Autodesk Inventor part; units mm, degrees
ref_plane "YZ Plane" through (0, 0, 0) normal (1, 0, 0) x (0, 1, 0)
ref_plane "XZ Plane" through (0, 0, 0) normal (0, 1, 0) x (-1, 0, 0)
ref_plane "XY Plane" through (0, 0, 0) normal (0, 0, 1) x (1, 0, 0)
sketch "Sketch1" plane through (0, 0, 0) normal (0, 0, 1) x (1, 0, 0)
  arc A0 (967.6192, 924.0732) -> (967.7873, 1075.2272) centre (902.2196, 999.723) ccw
  arc A1 (983.2683, 893.0126) -> (983.4428, 1106.3006) centre (902.2196, 999.723) ccw
  line L0 (965.7611, 927.7614) -> (985.0977, 889.3816)
  line L1 (966.6908, 925.9161) -> (1011.6908, 925.9161) construction
  arc A2 (985.0977, 889.3816) -> (985.2727, 1109.9327) centre (902.2196, 999.723) ccw
  line L2 (965.9281, 1071.5369) -> (985.2727, 1109.9327)
  arc A3 (965.7611, 927.7614) -> (965.9281, 1071.5369) centre (902.2196, 999.723) ccw
  line L3 (977.4986, 940.149) -> (980.6353, 937.6667)
  point P0 (0, 0)
  point P1 (983.9681, 893.1)
  point P2 (990.6031, 1100.4422)
  point P3 (968.1775, 1074.8866)
  dimension "d28" = 100
  dimension "d33" = 63.26
  dimension "d34" = 4
  dimension "d40" = 4
  dimension "d41" = 4
extrude "Extrusion6" add sketch "Sketch1" along normal blind 5
extrude "Extrusion7" add sketch "Sketch1" along normal blind 17 contours L3 A3 L2 A0 | A1 L2 A2 L0
sketch "Sketch5" plane through (0, 0, 5) normal (0, 0, 1) x (1, 0, 0)
  arc A0 (965.7611, 927.7614) -> (977.4986, 940.149) centre (902.2196, 999.723) ccw
  line L0 (965.7611, 927.7614) -> (970.2605, 918.8308)
  line L1 (965.7611, 927.7614) -> (983.2683, 893.0126)
  line L2 (977.4986, 940.149) -> (985.1361, 933.6938)
  arc A1 (965.7611, 927.7614) -> (977.4986, 940.149) centre (902.2196, 999.723) ccw
  arc A2 (965.7611, 927.7614) -> (974.9009, 937.006) centre (902.2196, 999.723) ccw
  line L3 (974.9009, 937.006) -> (982.5384, 930.5509)
  arc A3 (970.2605, 918.8308) -> (982.5384, 930.5509) centre (950.8165, 951.4915) ccw
  point P0 (0, 0)
  dimension "d42" = 10
  dimension "d43" = 10
  dimension "d46" = 13
  dimension "d47" = 10
extrude "Extrusion8" cut sketch "Sketch5" along normal through all both and the other way through all
sketch "Sketch6" plane through (0, 0, 5) normal (0, 0, 1) x (1, 0, 0)
  arc A0 (974.9009, 937.006) -> (965.9281, 1071.5369) centre (902.2196, 999.723) ccw
  arc A1 (985.0977, 889.3816) -> (985.2727, 1109.9327) centre (902.2196, 999.723) ccw
  line L0 (985.8441, 1046.8712) -> (1027.8759, 1046.8712) construction
  line L1 (985.2727, 1109.9327) -> (965.9281, 1071.5369)
  line L2 (965.9281, 1071.5369) -> (985.2727, 1109.9327)
  arc A2 (985.8441, 1046.8712) -> (965.9281, 1071.5369) centre (902.2196, 999.723) ccw
  arc A3 (1007.3627, 1089.1038) -> (985.2727, 1109.9327) centre (902.2196, 999.723) ccw
  line L3 (985.8441, 1046.8712) -> (1007.3627, 1089.1038)
  point P0 (0, 0)
  dimension "d51" = 63
extrude "Extrusion9" cut sketch "Sketch6" along normal through all both and the other way through all
sketch "Sketch7" plane through (0, 0, 5) normal (0, 0, 1) x (1, 0, 0)
  arc A0 (977.4782, 940.1232) -> (985.8441, 1046.8712) centre (902.2196, 999.723) ccw
  arc A1 (980.614, 937.6399) -> (988.005, 1051.1123) centre (902.2196, 999.723) ccw
  arc A2 (974.9009, 937.006) -> (985.8441, 1046.8712) centre (902.2196, 999.723) ccw
  line L0 (985.8441, 1046.8712) -> (988.005, 1051.1123)
  line L1 (985.8441, 1046.8712) -> (1007.3627, 1089.1038)
  line L2 (993.2753, 1030.1346) -> (996.6034, 1032.7639)
  point P0 (0, 0)
  dimension "d52" = 4
extrude "Extrusion10" cut sketch "Sketch7" along normal through all both and the other way through all
sketch "Sketch8" plane through (0, 0, 17) normal (0, 0, 1) x (1, 0, 0)
  arc A0 (983.2683, 893.0126) -> (1005.3901, 1085.2324) centre (902.2196, 999.723) ccw
  arc A1 (1014.3006, 1073.1658) -> (1005.3901, 1085.2324) centre (902.2196, 999.723) ccw
  line L0 (988.005, 1051.1123) -> (1007.3627, 1089.1038)
  line L1 (1005.3901, 1085.2324) -> (1007.3627, 1089.1038)
  line L2 (1014.3006, 1073.1658) -> (1017.6463, 1075.3581)
  arc A2 (985.0977, 889.3816) -> (1007.3627, 1089.1038) centre (902.2196, 999.723) ccw
  arc A3 (1017.6463, 1075.3581) -> (1007.3627, 1089.1038) centre (902.2196, 999.723) ccw
  point P0 (0, 0)
  dimension "d55" = 15
  dimension "d56" = 4
  dimension "d57" = 138
extrude "Extrusion11" cut sketch "Sketch8" against normal blind 12
sketch "Sketch10" plane through (0, 0, 5) normal (0, 0, 1) x (1, 0, 0)
  line L0 (993.2753, 1030.1346) -> (996.6034, 1032.7639)
  arc A0 (996.6034, 1032.7639) -> (988.005, 1051.1123) centre (902.2196, 999.723) ccw
  line L1 (988.005, 1051.1123) -> (1007.3627, 1089.1038)
  arc A1 (1017.6463, 1075.3581) -> (1007.3627, 1089.1038) centre (902.2196, 999.723) ccw
  line L2 (1014.3006, 1073.1658) -> (1017.6463, 1075.3581)
  arc A2 (983.2683, 893.0126) -> (1014.3006, 1073.1658) centre (902.2196, 999.723) ccw
  line L3 (983.2683, 893.0126) -> (970.2605, 918.8308)
  arc A3 (970.2605, 918.8308) -> (982.5384, 930.5509) centre (950.8165, 951.4915) ccw
  line L4 (982.5384, 930.5509) -> (974.9009, 937.006)
  arc A4 (974.9009, 937.006) -> (977.4986, 940.149) centre (902.2196, 999.723) ccw
  arc A5 (977.4986, 940.149) -> (993.2753, 1030.1346) centre (902.2196, 999.723) ccw
  arc A6 (980.6353, 937.6667) -> (996.6034, 1032.7639) centre (902.2196, 999.723) ccw
  line L5 (977.4986, 940.149) -> (980.6353, 937.6667)
  arc A7 (985.0977, 889.3816) -> (1017.6463, 1075.3581) centre (902.2196, 999.723) ccw
  line L6 (985.0977, 889.3816) -> (983.2683, 893.0126)
  line L7 (970.2605, 918.8308) -> (988.005, 1051.1123)
  line L8 (977.3926, 1032.2651) -> (974.8751, 1035.6786)
  arc A8 (988.005, 1051.1123) -> (974.8751, 1035.6786) centre (1057.2145, 978.9317) ccw
  line L9 (988.005, 1051.1123) -> (979.3441, 1092.8623)
  arc A9 (979.3441, 1092.8623) -> (965.8014, 1082.3127) centre (1057.2145, 978.9317) ccw
  line L10 (968.4511, 1079.3162) -> (965.8014, 1082.3127)
  arc A10 (973.7155, 1083.7358) -> (945.5606, 904.8412) centre (1057.2145, 978.9317) ccw
  line L11 (950.9084, 897.3534) -> (970.2605, 918.8308)
  arc A11 (961.5054, 933.3723) -> (970.2605, 918.8308) centre (997.6246, 945.2125) ccw
  line L12 (961.5054, 933.3723) -> (970.5741, 937.5864)
  arc A12 (968.8965, 941.3029) -> (970.5741, 937.5864) centre (1057.2145, 978.9317) ccw
  arc A13 (977.3926, 1032.2651) -> (968.8965, 941.3029) centre (1057.2145, 978.9317) ccw
  arc A14 (974.8751, 1035.6786) -> (965.2166, 939.735) centre (1057.2145, 978.9317) ccw
  line L13 (968.8965, 941.3029) -> (965.2166, 939.735)
  arc A15 (965.8014, 1082.3127) -> (948.1868, 894.3329) centre (1057.2145, 978.9317) ccw
  line L14 (948.1868, 894.3329) -> (950.9084, 897.3534)
  line L15 (970.2605, 918.8308) -> (948.1868, 894.3329)
  line L16 (970.2605, 918.8308) -> (985.0977, 889.3816)
  line L17 (985.0977, 889.3816) -> (975.4208, 817.2429)
  line L18 (948.1868, 894.3329) -> (938.5099, 822.1942)
  line L19 (945.5606, 904.8412) -> (934.5454, 822.726)
  line L20 (934.5454, 822.726) -> (979.3853, 816.7111)
  line L21 (979.3853, 816.7111) -> (990.4004, 898.8263)
  line L22 (945.5606, 904.8412) -> (948.1868, 894.3329)
  line L23 (985.0977, 889.3816) -> (990.4004, 898.8263)
  line L24 (988.005, 1051.1123) -> (1007.3627, 1089.1038)
  line L25 (988.005, 1051.1123) -> (979.3441, 1092.8623)
  line L26 (988.005, 1051.1123) -> (1007.3627, 1089.1038)
  line L27 (978.9999, 1153.216) -> (1023.6004, 1147.2332)
  line L28 (970.2605, 918.8308) -> (988.005, 1051.1123)
  line L29 (978.9999, 1153.216) -> (969.9631, 1085.8484)
  line L30 (1023.6004, 1147.2332) -> (1014.5636, 1079.8656)
  line L31 (973.7155, 1083.7358) -> (982.9644, 1152.6842)
  line L32 (1019.6359, 1147.765) -> (1010.3871, 1078.8166)
  arc A16 (990.4004, 898.8263) -> (1010.3871, 1078.8166) centre (902.2196, 999.723) ccw
  arc A17 (996.6034, 1032.7639) -> (988.005, 1051.1123) centre (902.2196, 999.723) ccw
  arc A18 (996.6034, 1032.7639) -> (988.005, 1051.1123) centre (902.2196, 999.723) ccw
  arc A19 (1000.3787, 1034.0856) -> (990.1322, 1055.2871) centre (902.2196, 999.723) ccw
  line L33 (993.2753, 1030.1346) -> (999.9157, 1035.3808)
  line L34 (988.005, 1051.1123) -> (990.1322, 1055.2871)
  arc A20 (988.005, 1051.1123) -> (974.8751, 1035.6786) centre (1057.2145, 978.9317) ccw
  line L35 (988.005, 1051.1123) -> (979.3441, 1092.8623)
  arc A21 (987.0533, 1055.7001) -> (971.5815, 1037.9485) centre (1057.2145, 978.9317) ccw
  line L36 (977.3926, 1032.2651) -> (972.3695, 1039.0759)
  point P0 (0, 0)
  point P1 (982.4326, 1148.7197)
  point P2 (1018.8217, 1141.6953)
  point P3 (980.2267, 1088.6079)
  point P4 (1005.3901, 1085.2324)
  point P5 (1011.1435, 1084.4555)
  point P6 (944.768, 898.933)
  point P7 (989.6079, 892.9181)
  point P8 (1001.3002, 1150.2246)
  point P9 (956.9654, 819.7185)
  dimension "d60" = 132.2815
  dimension "d61" = 4
  dimension "d62" = 4
  dimension "d64" = 45
  dimension "d65" = 22.5
  dimension "d66" = 4
  dimension "d74" = 100
  dimension "d75" = 100
  dimension "d76" = 4
extrude "Extrusion12" add sketch "Sketch10" against normal blind 5 contours L9 A9 L31 L27 L32 A1 L1 | A8 L36 A21 L9 | L3 L6 L17 L20 L18 L14 L11 | L11 L14 L22 A10 L31 A9 L9 A21 L36 A14 L13 A12 L12 A11
extrude "Extrusion13" add sketch "Sketch10" along normal blind 12 and the other way blind 5 contours L8 A13 L13 A14 | L32 L27 L30 A1 | A1 L2 A16 L32 | A7 L21 L20 L17 | L18 L20 L19 A15 | A15 L19 L22 | L31 A10 L10 A9 | A9 L29 L27 L31 | A15 L10 A10 L19
extrude "Extrusion14" cut sketch "Sketch10" against normal blind 12 contours A0 L1 A19 L33 | A8 L36 A21 L9
properties part number "outside3"
Design review of the part built by this model. Coordinates are the model's own, in mm. A direction names the side the tool comes from. Coordinates: 2 decimals unless noted, no trailing zeros. Write each loop counter-clockwise with the first axis right and the second up, starting at its lowest first coordinate (ties: lowest second). Pieces come first, ordered by that corner, then holes. Notation, with made-up numbers: (-6.75, 77) -> (48.25, 77) arc R17 ccw to (48.25, 99) -> close; hole circle Ø7 at (7.5, 73). An arc over 180 degrees is marked (long way). Write each question's results on one line, items separated by ' | '. Start each with the question number.
(1) Take a section at B-B on z = 9.5. Give the number of separate pieces and of enclosed holes in the cut face, and give its area (3 significant figures).
(2) For line 1 along X through (y, z) = (985, 13.25); line 2 along X through (y, z) = (960, 15.25); line 3 along Z through (x, y) = (950, 906), list the stretches that pass through material, from the lowest coordinate up. Write a range as from..to.
(3) Take a section at C-C on y = 1094. Write out the cut boundary in (x, z).
(4) Clearance check with flat-ended pins moving along their axes: P1, Ø2, axis at x = 995, z = 5.5, coming from the -Y side; P2, Ø10, axis at y = 853.5, z = 8, coming from the +X side. State where each tip first meets the part, or that it passes through.
(5) The part is to be moulded in two halves that separate along Y. For faces 1 (the face through (961, 984, 17)), 2 (the face through (978.275, 1117.727, 10.916)), 3 (the face through (956.65, 819.76, 4.84)), 4 (the face through (939.728, 861.363, 8.381)), say which applies: pulls with the +Y half, pulls with the -Y half, needs draft (parallel to the pull), parting line crosses it, or undercut.
(6) Tool access review of faces 5 (the face through (923, 988, 17)), 6 (the face through (946.855, 899.661, 10.916)), 7 (the face through (978.67, 933.82, 2.46)): name each direction out of +Z, -Z, +X, -X, +Y, -Y from which nothing blocks a thin tool from reaching the whole face with its end or side.
(7) Take a section at A-A on y = 1021. Write out the cut boundary in (x, z), and give its area (3 significant figures).
Results found:
1) separate pieces: 4 | enclosed holes: 0 | area: 3,600 mm2
2) line 1: x = 919.35..923.35, 957.4..961.41, 997.08..1001.13, 1035.41..1039.43 | line 2: x = 920.52..924.56, 959.02..963.1, 989.62..993.99, 1030.2..1034.38 | line 3: z = 0..5
3) outline: (971.06, 0) -> (1016.46, 0) -> (1016.46, 17) -> (1012.42, 17) -> (1012.42, 5) -> (975.09, 5) -> (975.09, 17) -> (971.06, 17) -> close
4) P1: stops at y = 896.67 | P2: stops at x = 984.99
5) face 1: needs draft | face 2: undercut | face 3: pulls with the -Y half | face 4: undercut
6) face 5: +Z, +X, -X, +Y, -Y | face 6: +Z | face 7: +Z, -Z
7) outline: (925.78, 0) -> (970.92, 0) -> (970.92, 17) -> (966.49, 17) -> (966.49, 5) -> (929.99, 5) -> (929.99, 17) -> (925.78, 17) -> close; (995.83, 0) -> (1038.57, 0) -> (1038.57, 17) -> (1034.52, 17) -> (1034.52, 5) -> (999.93, 5) -> (999.93, 17) -> (995.83, 17) -> close | area: 641 mm2
